Input: part model. Units: mm. Frame: model coordinates. Face numbers are marked on the shaded views. A direction names the side the tool comes from. Give positions to 0.01 mm unless a question says otherwise; leave off trailing zeros. Order: outer loops, then holes, each group sorted by start corner. A loop starts at its lowest first (then second) coordinate and runs counter-clockwise, first axis right, second up. Notation, with made-up numbers: (-24.75, -7) -> (31.25, -7) arc R14 ccw to (31.25, -1) -> close; hole circle Ø7 at (14.25, -1.5). An arc over 180 degrees is marked (long way). Use a Markdown table: item, result. Add a question column.
Autodesk Inventor part; units mm, degrees
ref_plane "YZ Plane" through (0, 0, 0) normal (1, 0, 0) x (0, 1, 0)
ref_plane "XZ Plane" through (0, 0, 0) normal (0, 1, 0) x (-1, 0, 0)
ref_plane "XY Plane" through (0, 0, 0) normal (0, 0, 1) x (1, 0, 0)
ref_plane "РабПлоскость1" through (0, 0, 0) normal (0, 0, 1) x (1, 0, 0)
sketch "Эскиз1" plane through (0, 0, 0) normal (0, 0, 1) x (1, 0, 0)
  line L0 (-70, -92) -> (-70, 92)
  line L1 (-62, 100) -> (62, 100)
  line L2 (70, 92) -> (70, -92)
  line L3 (62, -100) -> (-62, -100)
  line L4 (-70, -100) -> (70, 100) construction
  line L5 (-70, 100) -> (70, -100) construction
  arc A0 (-62, 100) -> (-70, 92) centre (-62, 92) ccw
  arc A1 (-70, -92) -> (-62, -100) centre (-62, -92) ccw
  arc A2 (62, -100) -> (70, -92) centre (62, -92) ccw
  arc A3 (70, 92) -> (62, 100) centre (62, 92) ccw
  line L6 (0, 75) -> (-40, 75)
  line L7 (-40, 75) -> (40, 75)
  line L8 (40, 75) -> (40, -75)
  line L9 (40, -75) -> (-40, -75)
  line L10 (-40, -75) -> (-40, 75)
  circle A4 centre (-40, 75) radius 11
  circle A5 centre (40, 75) radius 11
  circle A6 centre (-40, -75) radius 11
  circle A7 centre (40, -75) radius 11
  point P0 (0, 0)
  point P1 (0, 0)
  dimension "d24" = 200
  dimension "d25" = 140
  dimension "d26" = 8
  dimension "d27" = 8
  dimension "d28" = 8
  dimension "d29" = 8
  dimension "d31" = 40
  dimension "d32" = 80
  dimension "d33" = 150
  dimension "d34" = 22
  dimension "d35" = 22
  dimension "d36" = 22
  dimension "d37" = 22
extrude "Выдавливание1" add sketch "Эскиз1" along normal blind 50 contours L0 A0 L1 A3 L2 A2 L3 A1 | L7 A5 L8 A7 L9 A6 L10 A4 L6
sketch "Эскиз2" plane through (0, 0, 0) normal (0, 0, -1) x (-1, 0, 0)
  circle A0 centre (0, 0) radius 50
  dimension "d2" = 100
extrude "Выдавливание2" add sketch "Эскиз2" along normal blind 15
sketch "Эскиз3" plane through (0, 0, 50) normal (0, 0, 1) x (1, 0, 0)
  circle A0 centre (0, 0) radius 45
  dimension "d5" = 90
extrude "Выдавливание3" add sketch "Эскиз3" along normal blind 25
fillet "Сопряжение1" radius 10 1 edges at (-45, 0, 50)
sketch "Эскиз4" plane through (0, 0, 75) normal (0, 0, 1) x (1, 0, 0)
  circle A0 centre (0, 0) radius 55
  circle A1 centre (0, 0) radius 22.5
  dimension "d9" = 45
extrude "Выдавливание4" cut sketch "Эскиз4" against normal through all contours A1
chamfer "Фаска1" distance 2 angle 45 3 edges at (-22.5, 0, 75) (50, 0, -15) (-22.5, 0, -15)
sketch "Эскиз5" plane through (0, 0, 0) normal (1, 0, 0) x (0, 1, 0)
  line L0 (-24.5, -15) -> (24.5, -15)
  line L1 (48, -15) -> (-48, -15)
  line L2 (22.5, 73) -> (22.5, -13)
  line L3 (22.5, -15) -> (22.5, -8)
  line L4 (22.5, -8) -> (27.5, -8)
  line L5 (27.5, -8) -> (29.3756, -15)
  line L6 (0, -32.6) -> (0, 90.6)
  point P0 (0, 0)
  dimension "d15" = 7
  dimension "d16" = 5
  dimension "d17" = 105
revolve "Вращение1" cut sketch "Эскиз5" angle 360 about axis through (0, 0, -10) along (0, 0, 1)
chamfer "Фаска2" distance 2 angle 45 1 edges at (-22.5, 0, -8)
fillet "Сопряжение2" radius 8 8 edges at (67.6569, 97.6569, 50) (0, 100, 50) (-67.6569, 97.6569, 50) (-70, 0, 50) (-67.6569, -97.6569, 50) (0, -100, 50) (67.6569, -97.6569, 50) (70, 0, 50)
properties part number "Фланецгайка_CPY" material "Сталь, углеродистая"
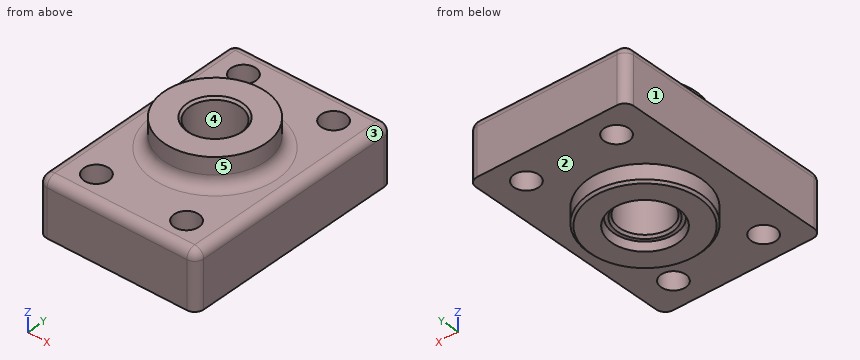
Q1. Section query C-C (z = 15). Return loops of the section in (x, y).
Q2. Draft query along Y for the marked faces 3, 4 and 5. Return one class per face: +Y half, -Y half, draft (parallel to the pull), parting line (faces both ways), or undercut.
Q3. Section query D-D (y = -75). Return loops of the section in (x, z).
Q4. Access query for the marked faces 1 and 2. Directions: +Z, -Z, +X, -X, +Y, -Y. A direction counts if a zero-diameter tool reaches every point of the face in a straight line with its end or side. Return the directions, or none.
Q5. Ray query, line 1 (X direction, y = 75, z = 38.5); line 2 (Y direction, x = -40, z = 18); line 3 (Y direction, x = 0, z = 24.5). Return the intervals inside material, ascending.
Q6. First-contact query: pin 1 (17.5 mm diameter, centred on x = -40, y = 75, fed in from +Z); pin 2 (3 mm diameter, centred on y = 44.5, z = 46, fed in from +X); pin 3 (1 mm diameter, centred on x = -37.5, z = 43, fed in from -Y). Flat tips, straight axial feed; report the tip coordinate or a pass-through.
Solution:
| question | item | result |
|---|---|---|
| 1 | outline | (-70, -92) arc R8 ccw to (-62, -100) -> (62, -100) arc R8 ccw to (70, -92) -> (70, 92) arc R8 ccw to (62, 100) -> (-62, 100) arc R8 ccw to (-70, 92) -> close; hole circle Ø22 at (-40, -75); hole circle Ø22 at (-40, 75); hole circle Ø45 at (0, 0); hole circle Ø22 at (40, -75); hole circle Ø22 at (40, 75) |
| 2 | face 3 | draft |
| 2 | face 4 | undercut |
| 2 | face 5 | parting line |
| 3 | outline | (-70, 0) -> (-51, 0) -> (-51, 50) -> (-62, 50) arc R8 ccw to (-70, 42) -> close; (-29, 0) -> (29, 0) -> (29, 50) -> (-29, 50) -> close; (51, 0) -> (70, 0) -> (70, 42) arc R8 ccw to (62, 50) -> (51, 50) -> close |
| 4 | face 1 | +Z, -Z, -X, +Y, -Y |
| 4 | face 2 | -Z |
| 5 | line 1 | x = -70 to -51, -29 to 29, 51 to 70 |
| 5 | line 2 | y = -100 to -86, -64 to 64, 86 to 100 |
| 5 | line 3 | y = -100 to -22.5, 22.5 to 100 |
| 6 | pin 1 | passes through |
| 6 | pin 2 | stops at x = 69.6 |
| 6 | pin 3 | stops at y = -99.98 |
